Source: CAD feature listing. Evaluate the final solid. Frame: model axes, mm. A direction names the side the tool comes from. Give positions to 0.01 mm unless a question says otherwise; leave off trailing zeros. Order: outer loops, then holes, each group sorted by start corner. A loop starts at its lowest first (then second) coordinate and runs counter-clockwise, first axis right, second up. Notation, with made-up numbers: M 26,-0.5 L 42,-0.5 A26 ccw 42,26.5 Z; hole C 37,61 d2. An arc over 180 degrees is marked long. Answer as a JSON object with one key per item and string values. Group by question number.
1. Pin query (flat end, axial travel): P1, Ø4, axis at x = -5.5, z = 8.5, coming from the +Y side; P2, Ø4, axis at y = -13.5, z = -0.5, coming from the -X side; P3, Ø3, axis at x = 2, y = -15.5, coming from the -Z side. Return the tip coordinate at first contact, or that it passes through.
2. Section query B-B (x = 0). Output: boundary loops of the cut face in (y, z), plus the area to 3 significant figures.
3. Section query D-D (y = -3). Output: boundary loops of the cut face in (x, z).
4. Set-up query: faces 1 (the cylindrical face through (1.617, -12.83, -0.67)), 2 (the flat face through (0, -17.9, 0)). Return all of +Z, -Z, +X, -X, +Y, -Y with unobstructed straight access to the full face (end or side cutting, diameter ignored); none if empty.
5. Section query C-C (y = -16.5). Output: boundary loops of the cut face in (x, z).
6. Section query A-A (z = 0). Output: boundary loops of the cut face in (x, y), plus the area to 3 significant figures.
7. Material intervals for L1, parallel to Y at x = 4.75, z = 4.75; L2, parallel to Y at x = 7.5, z = 6.75; L3, parallel to Y at x = -9.75, z = 5.25, sorted ascending. Write a range as [from, to].
from build123d import *

# Parameters (mm, degrees)
F0_R     = 11.5
F1_DEPTH = 7.9
F2_R     = 1.75
F3_DEPTH = 10
F4_R     = 3.95


with BuildPart() as f1:
    # F0 (on Front) → F1 (new body)
    with BuildSketch(Plane.XZ):
        Circle(F0_R)
    extrude(amount=F1_DEPTH)

    # F2 (on face) → F3 (join)
    with BuildSketch(Plane.XZ.offset(7.9)):
        Circle(F2_R)
    extrude(amount=F3_DEPTH)

    # F4 (on Right) → F5 (revolve, cut)
    with BuildSketch(Plane.YZ):
        with Locations((-3.95, 13)):
            Circle(F4_R)
    revolve(axis=Axis((0, -5.14938, 0), (0, 1, 0)), mode=Mode.SUBTRACT)


solid = f1.part
Answer sheet:
{
 "1": {"P1": "y = 0", "P2": "x = -1.75", "P3": "z = -1.68"},
 "2": {"outline": "M -17.9,-1.75 L -7.9,-1.75 L -7.9,-11.5 L -7.6,-11.5 A3.95 cw -0.3,-11.5 L 0,-11.5 L 0,11.5 L -0.3,11.5 A3.95 cw -7.6,11.5 L -7.9,11.5 L -7.9,1.75 L -17.9,1.75 Z", "area": "191 mm^2"},
 "3": {"outline": "C 0,0 d18.33"},
 "4": {"face 1": "-Y", "face 2": "+Z, -Z, +X, -X, -Y"},
 "5": {"outline": "C 0,0 d3.5"},
 "6": {"outline": "M -11.5,-7.9 L -1.75,-7.9 L -1.75,-17.9 L 1.75,-17.9 L 1.75,-7.9 L 11.5,-7.9 L 11.5,-7.6 A3.95 cw 11.5,-0.3 L 11.5,0 L -11.5,0 L -11.5,-0.3 A3.95 cw -11.5,-7.6 Z", "area": "191 mm^2"},
 "7": {"L1": "[-7.9, 0]", "L2": "[-7.9, -6.62], [-1.28, 0]", "L3": "[-7.9, -7.4], [-0.5, 0]"}
}
